from build123d import *

# Parameters (mm, degrees)
SKETCH1_R           = 2.413
BOSS_EXTRUDE1_DEPTH = 25.4
SKETCH3_W           = 2.413
SKETCH3_H           = 0.635
SKETCH4_W           = 14.174557954
SKETCH4_H           = 1.397
CUT_EXTRUDE1_DEPTH  = 1.016


with BuildPart() as part:
    # Sketch1 → Boss-Extrude1 (new body)
    with BuildSketch(Plane(origin=(0, 0, 0), x_dir=(1, 0, 0), z_dir=(0, 1, 0))):
        Circle(SKETCH1_R)
    extrude(amount=BOSS_EXTRUDE1_DEPTH)

    # Sketch2 → Revolve1 (revolve)
    with BuildSketch(Plane.XY):
        Polygon((0, 25.4), (4.6355, 25.4), (0, 20.067467248), align=None)
    revolve(axis=Axis((0, 20.067467248, 0), (0, 1, 0)))

    # Sketch3 → Cut-Revolve1 (revolve, cut)
    with BuildSketch(Plane.XY):
        Polygon((2.413, 0), (0, 0), (2.413, 4.179438599), align=None)
        with Locations((1.2065, -0.3175)):
            Rectangle(SKETCH3_W, SKETCH3_H)
    revolve(axis=Axis((0, 4.385214031, 0), (0, -1, 0)), mode=Mode.SUBTRACT)

    # Sketch4 → Cut-Extrude1 (cut)
    with BuildSketch(Plane(origin=(0, 25.4, 0), x_dir=(1, 0, 0), z_dir=(0, 1, 0))):
        Rectangle(SKETCH4_W, SKETCH4_H)
    extrude(amount=-CUT_EXTRUDE1_DEPTH, mode=Mode.SUBTRACT)


solid = part.part
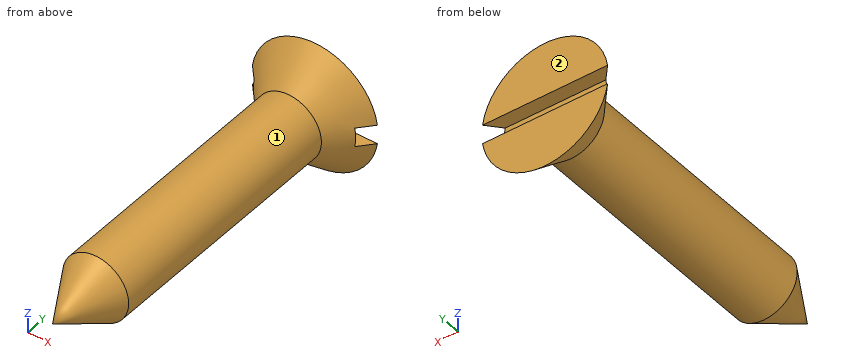
Geometry check sheet. Reference: the model listing, model coordinates, mm. Face numbers are marked on the shaded views. A direction names the side the tool comes from. Give positions to 0.01 mm unless a question says otherwise; leave off trailing zeros. Write each loop counter-clockwise with the first axis right and the second up, starting at its lowest first coordinate (ties: lowest second). Pieces come first, ordered by that corner, then holes.
1) Thickness scan on line 1 (Z direction, x = -0.25, y = 4); line 2 (Z direction, x = -1.75, y = 19.5); line 3 (Y direction, x = 1.25, z = -0.5). Record the ranges inside material, lowest first.
Values follow:
line 1: z = -2.3 to 2.3
line 2: z = -1.66 to 1.66
line 3: y = 2.33 to 24.38
2) Set-up check for the marked faces 1 and 2: record each of +Z, -Z, +X, -X, +Y, -Y from which the full face is reachable in a straight line by a thin tool's end or side.
Values follow:
face 1: -Y
face 2: +Z, -Z, +X, -X, +Y
3) Go/stop test with flat-tipped pins: pin 1 Ø1 at (x, y) = (-1, 11) entering from +Z; pin 2 Ø1.1 at (x, y) = (-0.5, 25) entering from +Z; pin 3 Ø2 at (y, z) = (21.5, -0.5) entering from +X; pin 4 Ø1.5 at (x, y) = (-3.5, 20.5) entering from -Z. Record where each tip stops, or that it passes through.
Values follow:
pin 1: stops at z = 2.36
pin 2: stops at z = 4.63
pin 3: stops at x = 2.41
pin 4: passes through
4) Cross-section at A-A (y = 15.75). Record the boundary of the cut face in (x, z), plus the area to 3 significant figures.
Values follow:
outline: circle Ø4.83 at (0, 0)
area: 18.3 mm2
